Here's the drawing with two shaded views (mm, measured from the low corner). I have some questions. Round coordinates to 2 decimals unless told otherwise and drop trailing zeros. Loops run counter-clockwise (first coordinate to the right, second up) from the corner with the lowest first, then second, coordinate; pieces in that order, holes last.
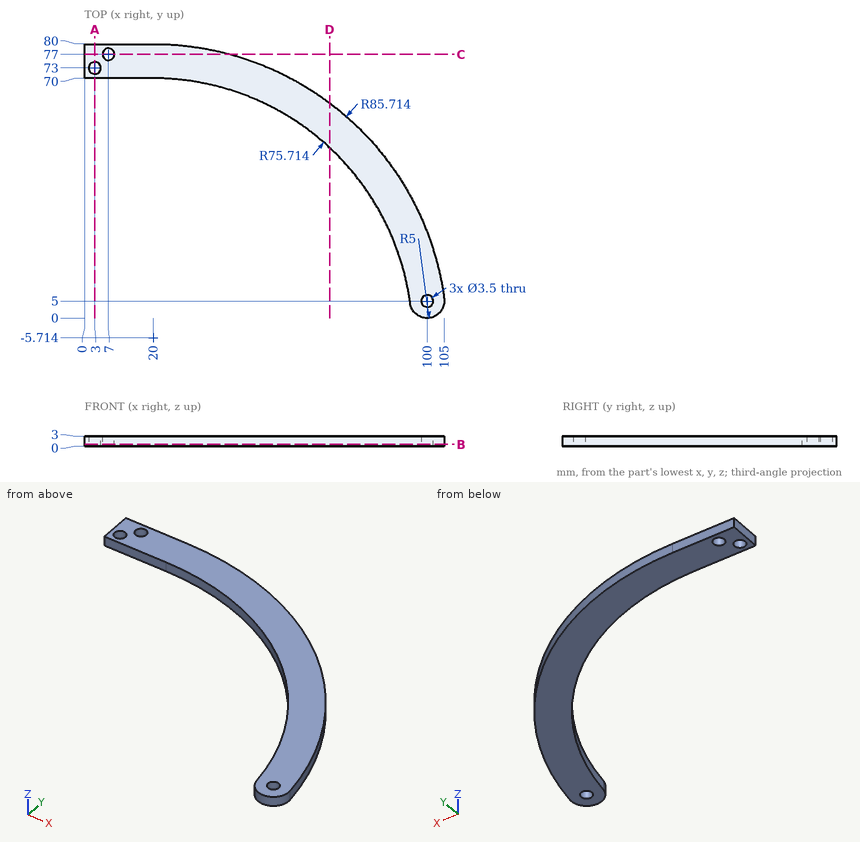
(1) If we section it at A-A, the plane x = 3: List the corners of the cut face in (y, z) for me.
Worked answers:
outline: (70, 0) - (71.25, 0) - (71.25, 3) - (70, 3) - close; (74.75, 0) - (80, 0) - (80, 3) - (74.75, 3) - close
(2) If we section it at B-B, the plane z = 0.6: List the corners of the cut face in (x, y) for me, then the cut area to 3 significant figures.
Worked answers:
outline: (0, 70) - (20, 70) arc R75.71 cw to (95.04, 4.34) arc R5 ccw to (104.96, 5.66) arc R85.71 ccw to (20, 80) - (0, 80) - close; hole circle Ø3.5 at (3, 73); hole circle Ø3.5 at (7, 77); hole circle Ø3.5 at (100, 5)
area: 1,370 mm2
(3) If I drill on line 1 (Y direction, x = 7, z = 1.9); line 2 (Y direction, x = 3, z = 2.1); line 3 (X direction, y = 5, z = 2.1), over which ranges is the centre line in solid material (lowest first)?
Worked answers:
line 1: y = 70 to 75.25, 78.75 to 80
line 2: y = 70 to 71.25, 74.75 to 80
line 3: x = 94.95 to 98.25, 101.75 to 105
(4) If we section it at D-D, the plane x = 71.5: List the corners of the cut face in (y, z) for me.
Worked answers:
outline: (49.79, 0) - (62.8, 0) - (62.8, 3) - (49.79, 3) - close
(5) Will this pin go through, and if not, where does the flat tip stop? P1, Ø1.5, axis at x = 6, z = 1.5, coming from the -Y side.
Worked answers:
P1: stops at y = 70
(6) If we section it at C-C, the plane y = 77: List the corners of the cut face in (x, z) for me, then the cut area to 3 significant figures.
Worked answers:
outline: (0, 0) - (5.25, 0) - (5.25, 3) - (0, 3) - close; (8.75, 0) - (42.48, 0) - (42.48, 3) - (8.75, 3) - close
area: 117 mm2
